from build123d import *

# Parameters (mm, degrees)
F0_W     = 600
F0_H     = 400
F1_DEPTH = 6
F2_W     = 600
F2_H     = 6
F2_H_2   = 5
F3_DEPTH = 25


with BuildPart() as f1:
    # F0 (on Top) → F1 (new body)
    with BuildSketch(Plane.XY):
        Rectangle(F0_W, F0_H)
    extrude(amount=F1_DEPTH)

    # F2 (on Top) → F3 (join)
    with BuildSketch(Plane.XY):
        with Locations((0, -132)):
            Rectangle(F2_W, F2_H)
        with Locations((0, -66.5)):
            Rectangle(F2_W, F2_H_2)
        with Locations((0, -1.5)):
            Rectangle(F2_W, F2_H_2)
        with Locations((0, 63.5)):
            Rectangle(F2_W, F2_H_2)
        with Locations((0, 128.5)):
            Rectangle(F2_W, F2_H_2)
        with Locations((0, -197.5)):
            Rectangle(F2_W, F2_H_2)
    extrude(amount=F3_DEPTH)


solid = f1.part
Source: CAD feature listing. Evaluate the final solid. Frame: model axes, mm. A direction names the side the tool comes from. Coordinates: 2 decimals unless noted, no trailing zeros. Loops run counter-clockwise (first coordinate to the right, second up) from the corner with the lowest first, then second, coordinate; pieces in that order, holes last. Notation, with made-up numbers: (6, -27.75) -> (54, -27.75) arc R11 cw to (54, -20.75) -> close; hole circle Ø5 at (7.5, 18). An arc over 180 degrees is marked (long way). Answer in a Markdown table with one row per item. Add a question column.
Q1. Contact query for flat-ended pins moving along their axis: pin 1 Ø3 at (x, z) = (-226.5, 21.5) entering from +Y; pin 2 Ø18 at (x, y) = (69.5, 32.5) entering from +Z. Output: stop coordinate, or through.
Q2. Section C-C on y = 150. Return the cut outline in (x, z), and give its area (3 significant figures).
Q3. Section A-A on z = 13.75. Return the cut outline in (x, y).
Q4. Section B-B on x = -16. Return the cut outline in (y, z), and give its area (3 significant figures).
Q5. Pull-direction query (Y, two-part tool) for faces 4 (the face through (-4, -64, 15)), 5 (the face through (-300, 42, 4)), 6 (the face through (-4, 131, 15)); classes: pulls with the +Y half, pulls with the -Y half, needs draft (parallel to the pull), parting line crosses it, or undercut.
Q6. Ray query, line 1 along Y through (x, z) = (-239.5, 8.25); line 2 along Z through (x, y) = (116.5, 146). Return the intervals inside material, ascending.
Q7. Reachability of faces 1 (the face through (-4, 166, 6)), 2 (the face through (300, 42, 4)), 3 (the face through (-4, 126, 15)) from +Z, -Z, +X, -X, +Y, -Y: full face, straight path, thin tool, end or side. Return the list, or none.
Computed values:
| question | item | result |
|---|---|---|
| 1 | pin 1 | stops at y = 131 |
| 1 | pin 2 | stops at z = 6 |
| 2 | outline | (-300, 0) -> (300, 0) -> (300, 6) -> (-300, 6) -> close |
| 2 | area | 3,600 mm^2 |
| 3 | outline | (-300, -200) -> (300, -200) -> (300, -195) -> (-300, -195) -> close; (-300, -135) -> (300, -135) -> (300, -129) -> (-300, -129) -> close; (-300, -69) -> (300, -69) -> (300, -64) -> (-300, -64) -> close; (-300, -4) -> (300, -4) -> (300, 1) -> (-300, 1) -> close; (-300, 61) -> (300, 61) -> (300, 66) -> (-300, 66) -> close; (-300, 126) -> (300, 126) -> (300, 131) -> (-300, 131) -> close |
| 4 | outline | (-200, 0) -> (200, 0) -> (200, 6) -> (131, 6) -> (131, 25) -> (126, 25) -> (126, 6) -> (66, 6) -> (66, 25) -> (61, 25) -> (61, 6) -> (1, 6) -> (1, 25) -> (-4, 25) -> (-4, 6) -> (-64, 6) -> (-64, 25) -> (-69, 25) -> (-69, 6) -> (-129, 6) -> (-129, 25) -> (-135, 25) -> (-135, 6) -> (-195, 6) -> (-195, 25) -> (-200, 25) -> close |
| 4 | area | 2,990 mm^2 |
| 5 | face 4 | undercut |
| 5 | face 5 | needs draft |
| 5 | face 6 | pulls with the +Y half |
| 6 | line 1 | y = -200 to -195, -135 to -129, -69 to -64, -4 to 1, 61 to 66, 126 to 131 |
| 6 | line 2 | z = 0 to 6 |
| 7 | face 1 | +Z, +X, -X, +Y |
| 7 | face 2 | +Z, -Z, +X, +Y, -Y |
| 7 | face 3 | +Z, +X, -X |
